The listing builds one solid part. Answer for the finished solid, in the listing's coordinates (mm). Face numbers are marked on the shaded views. A direction names the side the tool comes from. Coordinates: 2 decimals unless noted, no trailing zeros. Write each loop counter-clockwise with the first axis right and the second up, starting at its lowest first coordinate (ties: lowest second). Pieces come first, ordered by that corner, then holes.
(1) The part is cut by section B-B on x = 0. Determine the outline of the cut face in (y, z).
(2) The part is cut by section A-A on z = 0. Determine the outline of the cut face in (x, y), plus the area to 3 significant figures.
(3) The part is cut by section C-C on y = 20.75. Determine the outline of the cut face in (x, z), plus the area to 3 significant figures.
(4) Which of the six approach directions +Z, -Z, +X, -X, +Y, -Y give full straight-line access (tool end or side, diameter ignored) to the marked faces 1 and 2?
(5) Straight lines are drawn through the part: line 1 (Y direction, x = 0.1, z = 1.15); line 2 (X direction, y = 11.5, z = 1.3); line 3 (X direction, y = 7, z = -0.2). For each, find the intervals that lie inside material, in ascending order.
(6) The part is cut by section D-D on y = 8.25. Determine the outline of the cut face in (x, z) (1 decimal).
Autodesk Inventor part; units mm, degrees
ref_plane "YZ Plane" through (0, 0, 0) normal (1, 0, 0) x (0, 1, 0)
ref_plane "XZ Plane" through (0, 0, 0) normal (0, 1, 0) x (-1, 0, 0)
ref_plane "XY Plane" through (0, 0, 0) normal (0, 0, 1) x (1, 0, 0)
sketch "Sketch1" plane through (0, 0, 0) normal (0, 1, 0) x (-1, 0, 0)
  circle A0 centre (0, 0) radius 1.5875
  dimension "d0" = 3.175
extrude "Extrusion1" add sketch "Sketch1" along normal blind 19.05
thread "Thread1"
sketch "Sketch2" plane through (0, 19.05, 0) normal (0, 1, 0) x (1, 0, 0)
  circle A0 centre (0, 0) radius 1.0795
  dimension "d5" = 2.159
extrude "Extrusion2" add sketch "Sketch2" along normal blind 6.35
chamfer "Chamfer1" distance 0.254 angle 45 1 edges at (1.5875, 0, 0)
sketch "Sketch3" plane through (0, 0, 0) normal (1, 0, 0) x (0, 1, 0)
  point P0 (0, 0)
properties part number "burner_rod_1or3"
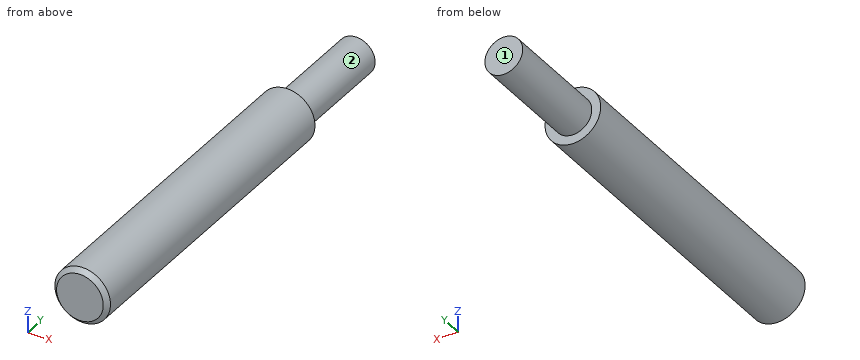
Model answer:
1. outline: (0, -1.33) - (0.25, -1.59) - (19.05, -1.59) - (19.05, -1.08) - (25.4, -1.08) - (25.4, 1.08) - (19.05, 1.08) - (19.05, 1.59) - (0.25, 1.59) - (0, 1.33) - close
2. outline: (-1.59, 0.25) - (-1.33, 0) - (1.33, 0) - (1.59, 0.25) - (1.59, 19.05) - (1.08, 19.05) - (1.08, 25.4) - (-1.08, 25.4) - (-1.08, 19.05) - (-1.59, 19.05) - close
2. area: 74.1 mm2
3. outline: circle Ø2.16 at (0, 0)
3. area: 3.66 mm2
4. face 1: +Z, -Z, +X, -X, +Y
4. face 2: +Y
5. line 1: y = 0 to 19.05
5. line 2: x = -0.91 to 0.91
5. line 3: x = -1.57 to 1.57
6. outline: circle Ø3.2 at (0, 0)
